Geometry: final body of the model. Coordinates: model frame, mm. Round coordinates to 2 decimals unless told otherwise and drop trailing zeros. Use CSV: the item, a comma, the result in double quotes.
from build123d import *

# Parameters (mm, degrees)
SKETCH1_W           = 210
SKETCH1_H           = 55
BOSS_EXTRUDE1_DEPTH = 3.175


with BuildPart() as part:
    # Sketch1 → Boss-Extrude1 (new body)
    with BuildSketch(Plane.XY):
        with Locations((-261.58829827, -18.441689147)):
            Rectangle(SKETCH1_W, SKETCH1_H)
        with BuildLine():
            Line((-183.826005128, -9.437626279), (-165.825906922, -9.437626279))
            Line((-165.825906922, -9.437626279), (-165.825906922, -27.359682536))
            Line((-165.825906922, -27.359682536), (-185.498112528, -27.359682536))
            add(Edge.make_bspline(
                [(-183.826005128, -9.437626279), (-184.381626607, -9.397687719), (-184.930515996, -9.424835034), (-186.015461991, -9.607009465), (-186.554689235, -9.764877403), (-187.316224975, -10.082704779), (-187.563814734, -10.202332624), (-188.04695947, -10.467917292), (-188.283591247, -10.614653216), (-188.967244505, -11.088099477), (-189.385834671, -11.445153232), (-190.155876141, -12.234064044), (-190.507940946, -12.668506087), (-191.124349263, -13.579620928), (-191.392257861, -14.05945224), (-191.73522916, -14.814675279), (-191.839717206, -15.072804389), (-192.025673908, -15.592230911), (-192.107659089, -15.854561779), (-192.321609275, -16.649175241), (-192.421750284, -17.189035513), (-192.508320777, -18.013979615), (-192.526449679, -18.291627862), (-192.540341709, -18.842430921), (-192.536260587, -19.116785649), (-192.490788714, -19.936695463), (-192.416446167, -20.47912245), (-192.234051872, -21.286034277), (-192.160881012, -21.555192562), (-191.992478644, -22.081128913), (-191.89721521, -22.338632762), (-191.57815234, -23.094708941), (-191.321465438, -23.577036127), (-190.86409563, -24.264793996), (-190.698255397, -24.489466796), (-190.347004112, -24.917221829), (-190.161879434, -25.120329067), (-189.577727686, -25.697021795), (-189.150303695, -26.038410046), (-188.444997142, -26.47773401), (-188.199013121, -26.611592551), (-187.699838217, -26.845624837), (-187.189859794, -27.048393537), (-186.658261328, -27.188597437), (-186.115554078, -27.296654363), (-185.837627103, -27.33444368), (-185.540644376, -27.356776903), (-185.519377345, -27.358278606), (-185.498112528, -27.359682536)],
                knots=[0, 0, 0, 0, 0.03125, 0.03125, 0.0625, 0.0625, 0.078125, 0.078125, 0.09375, 0.09375, 0.125, 0.125, 0.15625, 0.15625, 0.1875, 0.1875, 0.203125, 0.203125, 0.21875, 0.21875, 0.25, 0.25, 0.265625, 0.265625, 0.28125, 0.28125, 0.3125, 0.3125, 0.328125, 0.328125, 0.34375, 0.34375, 0.375, 0.375, 0.390625, 0.390625, 0.40625, 0.40625, 0.4375, 0.4375, 0.453125, 0.453125, 0.46875, 0.484375, 0.484375, 0.5, 0.5, 0.501205353, 0.501205353, 0.501205353, 0.501205353], degree=3))
        make_face(mode=Mode.SUBTRACT)
        with BuildLine():
            Line((-248.842639606, -9.34526812), (-230.842639606, -9.34526812))
            Line((-230.842639606, -9.34526812), (-230.842639606, -27.359569421))
            Line((-230.842639606, -27.359569421), (-248.122030426, -27.359569421))
            add(Edge.make_bspline(
                [(-248.842639606, -9.34526812), (-249.008492971, -9.34526812), (-249.174528912, -9.351217217), (-249.897892737, -9.403148293), (-250.439041218, -9.508791349), (-251.226902991, -9.764277117), (-251.486942339, -9.866389631), (-251.991898718, -10.100883467), (-252.478538383, -10.363667412), (-252.930635604, -10.679802053), (-253.365916766, -11.021909044), (-253.576181816, -11.207074635), (-254.170571266, -11.790206392), (-254.521054547, -12.216408682), (-254.984007031, -12.907063712), (-255.128207339, -13.146926319), (-255.391039985, -13.635131957), (-255.510280092, -13.884200022), (-255.833281599, -14.645561933), (-256.003111783, -15.174210606), (-256.250113173, -16.258400348), (-256.325565617, -16.804580713), (-256.371925399, -17.6295328), (-256.376170681, -17.905469832), (-256.362395823, -18.459237102), (-256.344221579, -18.737973637), (-256.257616038, -19.564249546), (-256.157308421, -20.105224546), (-255.942745346, -20.901816623), (-255.860495563, -21.164858437), (-255.673862588, -21.685807516), (-255.568906935, -21.944849427), (-255.224992289, -22.701497667), (-254.956918189, -23.181017599), (-254.49602176, -23.862551099), (-254.33253309, -24.083399995), (-253.984921716, -24.511848542), (-253.79988931, -24.720372449), (-253.217915831, -25.317918038), (-252.799712482, -25.674443478), (-252.12529242, -26.144005131), (-251.892576917, -26.289576641), (-251.410235402, -26.557308591), (-251.158897378, -26.680166876), (-250.389777098, -27.004646057), (-249.862976161, -27.161019247), (-249.050989853, -27.302657737), (-248.776672466, -27.334279323), (-248.37319776, -27.356189189), (-248.247527215, -27.359569421), (-248.122030426, -27.359569421)],
                knots=[0.990687447, 0.990687447, 0.990687447, 0.990687447, 1, 1, 1.03125, 1.03125, 1.046875, 1.046875, 1.0625, 1.078125, 1.078125, 1.09375, 1.09375, 1.125, 1.125, 1.140625, 1.140625, 1.15625, 1.15625, 1.1875, 1.1875, 1.21875, 1.21875, 1.234375, 1.234375, 1.25, 1.25, 1.28125, 1.28125, 1.296875, 1.296875, 1.3125, 1.3125, 1.34375, 1.34375, 1.359375, 1.359375, 1.375, 1.375, 1.40625, 1.40625, 1.421875, 1.421875, 1.4375, 1.4375, 1.46875, 1.46875, 1.484375, 1.484375, 1.491411882, 1.491411882, 1.491411882, 1.491411882], degree=3))
        make_face(mode=Mode.SUBTRACT)
    extrude(amount=BOSS_EXTRUDE1_DEPTH)


solid = part.part
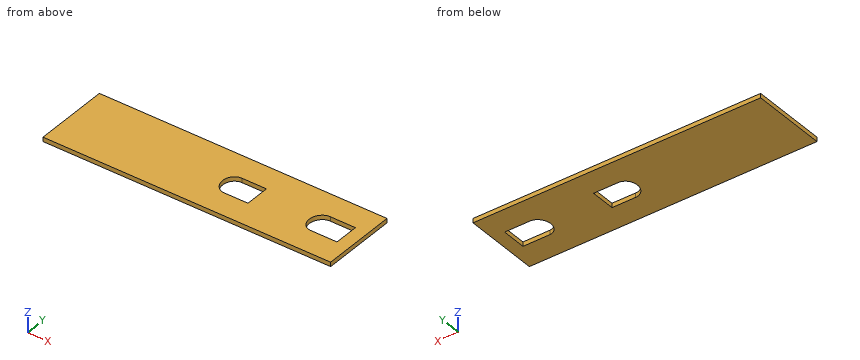
Item 1: Pin query (flat end, axial travel): P1, Ø2, axis at x = -323, y = -38, coming from the -Z side. Return the tip coordinate at first contact, or that it passes through.
Final values:
P1,"stops at z = 0"
Item 2: Section A-A on z = 0.8. Give the number of separate pieces and of enclosed holes in the cut face, plus the area to 3 significant figures.
Final values:
separate pieces,"1"
enclosed holes,"2"
area,"10,700 mm²"
Item 3: Material intervals for line 1 (X direction, y = -17, z = 2.55); line 2 (X direction, y = -19, z = 3); line 3 (Y direction, x = -166, z = 2.9), sorted ascending.
Final values:
line 1,"x = -366.59 to -256.33, -230.84 to -192.38, -165.83 to -156.59"
line 2,"x = -366.59 to -256.32, -230.84 to -192.54, -165.83 to -156.59"
line 3,"y = -45.94 to -27.36, -9.44 to 9.06"
